from build123d import *

# Parameters (mm, degrees)
SKETCH_R     = 27.25
PAD_DEPTH    = 4.1
SKETCH001_W  = 9
SKETCH001_H  = 9
POCKET_DEPTH = 5


with BuildPart() as part:
    # Sketch → Pad (new body)
    with BuildSketch(Plane.XY):
        Circle(SKETCH_R)
    extrude(amount=PAD_DEPTH)

    # Sketch001 (on DatumPlane) → Pocket (cut)
    with BuildSketch(Plane.XY.offset(4.1)):
        with Locations((0, 23.072699)):
            Rectangle(SKETCH001_W, SKETCH001_H)
    pocket = extrude(amount=-POCKET_DEPTH, mode=Mode.SUBTRACT)

    # Mirrored: Pocket across Sketch001 H_Axis
    add(pocket.mirror(Plane(origin=(0, 0, 4.1), x_dir=(0, 0, 1), z_dir=(0, 1, 0))), mode=Mode.SUBTRACT)


solid = part.part
Read the model definition and answer for the solid it produces. Units are mm, in the model's axes. A direction names the side the tool comes from. Coordinates: 2 decimals unless noted, no trailing zeros. Loops run counter-clockwise (first coordinate to the right, second up) from the corner with the lowest first, then second, coordinate; pieces in that order, holes last. Notation, with made-up numbers: (-8.5, 82.5) - (3.5, 82.5) arc R15 ccw to (3.5, 105.5) - close; hole circle Ø4 at (-27, 11.25). An arc over 180 degrees is marked (long way). Answer in a Markdown table with one row per item.
Q1. Straight lines are drawn through the part: line 1 along X through (y, z) = (-21, 3.25); line 2 along Y through (x, z) = (1.5, 1.9); line 3 along X through (y, z) = (-20.5, 0.5). For each, find the intervals that lie inside material, in ascending order. Write a range as [from, to].
Here are the results:
| item | result |
|---|---|
| line 1 | x = [-17.37, -4.5], [4.5, 17.37] |
| line 2 | y = [-18.57, 18.57] |
| line 3 | x = [-17.95, -4.5], [4.5, 17.95] |
Q2. Find section D-D on x = 3.5. Write down the section's boundary in (y, z), plus the area to 3 significant figures.
Here are the results:
| item | result |
|---|---|
| outline | (-18.57, 0) - (18.57, 0) - (18.57, 4.1) - (-18.57, 4.1) - close |
| area | 152 mm^2 |
Q3. Find section B-B on z = 2.9. Write down the section's boundary in (x, y), plus the area to 3 significant figures.
Here are the results:
| item | result |
|---|---|
| outline | (-4.5, -26.88) - (-4.5, -18.57) - (4.5, -18.57) - (4.5, -26.88) arc R27.25 ccw to (4.5, 26.88) - (4.5, 18.57) - (-4.5, 18.57) - (-4.5, 26.88) arc R27.25 ccw to start |
| area | 2,180 mm^2 |
Q4. Given P1, Ø2, axis at y = 24, z = 3, coming from the +X side; P2, Ø2, axis at x = -1, z = 3, coming from the +Y side; P3, Ø1.2, axis at y = 23.5, z = 2.5, coming from the -X side; P4, Ø8, axis at x = 15.5, y = 4.5, coming from the -Z side, each flat-ended and moving along its own axis, determine where each tip first touches the part or whether it passes through.
Here are the results:
| item | result |
|---|---|
| P1 | stops at x = 14.61 |
| P2 | stops at y = 18.57 |
| P3 | stops at x = -14.77 |
| P4 | stops at z = 0 |
Q5. For faces 1 (the flat face through (0, -18.573, 2)), 2 (the flat face through (0, 0, 4.1)), 3 (the flat face through (0, 18.573, 2)), determine the directions among +Z, -Z, +X, -X, +Y, -Y from which every point of the face is accessible in a straight line to the end or side of a thin tool.
Here are the results:
| item | result |
|---|---|
| face 1 | +Z, -Z, -Y |
| face 2 | +Z, +X, -X, +Y, -Y |
| face 3 | +Z, -Z, +Y |
Q6. Find section A-A on y = 20.5. Write down the section's boundary in (x, z).
Here are the results:
| item | result |
|---|---|
| outline | (-17.95, 0) - (-4.5, 0) - (-4.5, 4.1) - (-17.95, 4.1) - close; (4.5, 0) - (17.95, 0) - (17.95, 4.1) - (4.5, 4.1) - close |
Q7. Find section C-C on y = -23. Write down the section's boundary in (x, z), plus the area to 3 significant figures.
Here are the results:
| item | result |
|---|---|
| outline | (-14.61, 0) - (-4.5, 0) - (-4.5, 4.1) - (-14.61, 4.1) - close; (4.5, 0) - (14.61, 0) - (14.61, 4.1) - (4.5, 4.1) - close |
| area | 82.9 mm^2 |
